Check sheet for the modelled part. Datum: model origin and axes. Units: mm. A direction names the side the tool comes from. Coordinates: 2 decimals unless noted, no trailing zeros. Order: outer loops, then holes, each group sorted by start corner. A loop starts at its lowest first (then second) coordinate and runs counter-clockwise, first axis right, second up.
1. Gauge pin test, flat ends, axial feed: pin 1 Ø1 at (x, y) = (12, 3) entering from -Z; pin 2 Ø1.5 at (y, z) = (1.5, 65.5) entering from +X; pin 3 Ø2 at (y, z) = (1, 85.5) entering from +X; pin 4 Ø1 at (x, y) = (7.5, 2) entering from -Z. Record the tip position at first contact, or that the pin passes through.
2. Thickness scan on line 1 (Z direction, x = -3.5, y = 1.9); line 2 (Z direction, x = 9, y = 2.95) (3 decimals); line 3 (X direction, y = 3, z = 88.5). Record the ranges inside material, lowest first.
3. Cross-section at D-D (z = -3.5). Enter the section's corners in (x, y).
4. Draft check along X on faces 3 (the flat face through (17.5, 2, 32)), 4 (the cylindrical face through (-8.46, 0.99, 11.44)), 5 (the flat face through (0, 0, 28)). Enter one of: released by +X, released by -X, zero draft, split by the parting line, or undercut.
5. Cross-section at A-A (z = 79). Enter the section's corners in (x, y), then the cut area to 3 significant figures.
6. Set-up check for faces 1 (the flat face through (-13, 2, 63.5)), 2 (the cylindrical face through (13.343, 1.972, 76.324)): record each of +Z, -Z, +X, -X, +Y, -Y from which the full face is reachable in a straight line by a thin tool's end or side.
7. Cross-section at B-B (x = 0). Enter the section's corners in (y, z), then the cut area to 3 significant figures.
8. Cross-section at C-C (y = 3.25). Count the separate pieces of the cut face and the enclosed holes in it, then the cut area to 3 significant figures.
Autodesk Inventor part; units mm, degrees
ref_plane "YZ Plane" through (0, 0, 0) normal (1, 0, 0) x (0, 1, 0)
ref_plane "XZ Plane" through (0, 0, 0) normal (0, 1, 0) x (-1, 0, 0)
ref_plane "XY Plane" through (0, 0, 0) normal (0, 0, 1) x (1, 0, 0)
sketch "Esquisse3" plane through (0, 0, 0) normal (0, 1, 0) x (-1, 0, 0)
  line L0 (-6.5, 6.5) -> (6.5, 6.5) construction
  line L1 (6.5, 6.5) -> (6.5, -6.5) construction
  line L2 (6.5, -6.5) -> (-6.5, -6.5) construction
  line L3 (-6.5, -6.5) -> (-6.5, 6.5) construction
  line L4 (-6.5, 6.5) -> (6.5, -6.5) construction
  line L5 (6.5, 6.5) -> (-6.5, -6.5) construction
  line L6 (-11.5, 11.5) -> (11.5, 11.5) construction
  line L7 (11.5, 11.5) -> (11.5, -11.5) construction
  line L8 (11.5, -11.5) -> (-11.5, -11.5) construction
  line L9 (-11.5, -11.5) -> (-11.5, 11.5) construction
  line L10 (-11.5, 11.5) -> (11.5, -11.5) construction
  line L11 (11.5, 11.5) -> (-11.5, -11.5) construction
  line L12 (-6.5, 6.5) -> (-11.5, 6.5) construction
  line L13 (-11.5, 6.5) -> (-11.5, 11.5) construction
  line L14 (-11.5, 11.5) -> (-6.5, 11.5) construction
  line L15 (-6.5, 11.5) -> (-6.5, 6.5) construction
  line L16 (-6.5, -6.5) -> (-11.5, -6.5) construction
  line L17 (-11.5, -6.5) -> (-11.5, -11.5) construction
  line L18 (-11.5, -11.5) -> (-6.5, -11.5) construction
  line L19 (-6.5, -11.5) -> (-6.5, -6.5) construction
  line L20 (6.5, -6.5) -> (11.5, -6.5) construction
  line L21 (11.5, -6.5) -> (11.5, -11.5) construction
  line L22 (11.5, -11.5) -> (6.5, -11.5) construction
  line L23 (6.5, -11.5) -> (6.5, -6.5) construction
  line L24 (11.5, 11.5) -> (6.5, 11.5) construction
  line L25 (6.5, 11.5) -> (6.5, 6.5) construction
  line L26 (6.5, 6.5) -> (11.5, 6.5) construction
  line L27 (11.5, 6.5) -> (11.5, 11.5) construction
  circle A0 centre (9, 9) radius 2.5
  circle A1 centre (9, -9) radius 2.5
  circle A2 centre (-9, -9) radius 2.5
  circle A3 centre (-9, 9) radius 2.5
  circle A4 centre (0, 0) radius 17.5
  circle A5 centre (0, 0) radius 8.5
  line L28 (17.5, 0) -> (17.5, 65)
  line L29 (-17.5, 0) -> (-17.5, 65)
  line L30 (0, -17.5) -> (0, 82.5) construction
  circle A6 centre (0, 65) radius 17.5
  circle A7 centre (0, 65) radius 10
  line L31 (1.5, 74.8869) -> (-1.5, 74.8869)
  line L32 (-1.5, 74.8869) -> (-1.5, 97.3869)
  line L33 (-1.5, 97.3869) -> (1.5, 97.3869)
  line L34 (1.5, 97.3869) -> (1.5, 74.8869)
  line L35 (-2.5, 98.3869) -> (-2.5, 73.8869)
  line L36 (-2.5, 73.8869) -> (2.5, 73.8869)
  line L37 (2.5, 73.8869) -> (2.5, 98.3869)
  line L38 (2.5, 98.3869) -> (-2.5, 98.3869)
  line L39 (15.8869, 63.5) -> (9.8869, 63.5)
  line L40 (9.8869, 63.5) -> (9.8869, 66.5)
  line L41 (9.8869, 66.5) -> (15.8869, 66.5)
  line L42 (15.8869, 66.5) -> (15.8869, 63.5)
  point P0 (17.5, 63.5)
  point P1 (17.4356, 66.5)
  point P2 (2.5, 82.3205)
  point P3 (-2.5, 82.3205)
  point P4 (1.5, 82.4356)
  point P5 (-1.5, 82.4356)
  point P6 (-2.5, 74.6825)
  point P7 (2.5, 74.6825)
  dimension "d1" = 13
  dimension "d2" = 13
  dimension "d3" = 5
  dimension "d4" = 35
  dimension "d9" = 9
  dimension "d29" = 100
  dimension "d31" = 35
  dimension "d32" = 20
  dimension "d33" = 3
  dimension "d34" = 22.5
  dimension "d36" = 1
  dimension "d37" = 3
  dimension "d51" = 6
extrude "Extrusion1" add sketch "Esquisse3" along normal blind 4 contours A4 | A4 L29 A6 L28 | A6 L35 A7 L39 L42 L41 L37 | L37 A7 L34 A6 | A6 L34 L33 L32 L35 L38 L37 | A6 L32 A7 L35
chamfer "Chanfrein5" distance 1 distance2 2 1 edges at (11.5, 4, -9) measured on face at (0.0538, 4, 25.8921)
chamfer "Chanfrein6" distance 1 distance2 2 1 edges at (-6.5, 4, -9) measured on face at (0.0538, 4, 25.8921)
chamfer "Chanfrein7" distance 1 distance2 2 1 edges at (-6.5, 4, 9) measured on face at (0.0538, 4, 25.8921)
chamfer "Chanfrein8" distance 1 distance2 2 1 edges at (11.5, 4, 9) measured on face at (0.172, 4, 26.2038)
properties part number "Pièce_moteur_maintient_test_4"
Data:
1. pin 1: stops at z = -13.19
1. pin 2: stops at x = 17.5
1. pin 3: stops at x = 2.5
1. pin 4: stops at z = -16.04
2. line 1: z = -17.15 to -7.75, 7.75 to 55.63, 74.37 to 82.15
2. line 2: z = -15.008 to -11.975, -6.025 to 6.025, 11.975 to 60.641, 69.359 to 80.008
2. line 3: x = -2.5 to -1.5, 1.5 to 2.5
3. outline: (-17.15, 0) - (-7.75, 0) - (-7.75, 4) - (-17.15, 4) - close; (7.75, 0) - (17.15, 0) - (17.15, 4) - (7.75, 4) - close
4. face 3: released by +X
4. face 4: undercut
4. face 5: zero draft
5. outline: (-10.5, 0) - (-1.5, 0) - (-1.5, 4) - (-10.5, 4) - close; (1.5, 0) - (10.5, 0) - (10.5, 4) - (1.5, 4) - close
5. area: 72.0 mm2
6. face 1: +Y, -Y
6. face 2: +Z, +X, +Y, -Y
7. outline: (0, -17.5) - (4, -17.5) - (4, -8.5) - (0, -8.5) - close; (0, 8.5) - (4, 8.5) - (4, 55) - (0, 55) - close; (0, 97.39) - (4, 97.39) - (4, 98.39) - (0, 98.39) - close
7. area: 226 mm2
8. separate pieces: 1
8. enclosed holes: 6
8. area: 2,570 mm2
